Drawing for the job (mm, zero at the part's lowest x, y, z). A direction names the side the tool comes from. Round coordinates to 2 decimals unless told otherwise and drop trailing zeros. Write each loop counter-clockwise with the first axis right and the second up, starting at its lowest first coordinate (ties: lowest second). Pieces come first, ordered by that corner, then holes. Notation, with made-up numbers: M -13.5,48 L 20.5,48 A17 ccw 20.5,73 Z; hole C -5.5,-21 d1. An arc over 180 degrees is marked long. Use a Markdown table: item, result. Add a question column.
1) Slice it at A-A on x = 203. Write the cut outline in (y, z), plus the area to 3 significant figures.
2) Slice it at C-C on y = 90. Write the cut outline in (x, z), plus the area to 3 significant figures.
3) Two-plate mould, pull along Y, no slides. Class the marked faces 1, 2, 3 and 4: released by +Y, released by -Y, zero draft, split by the parting line, or undercut.
4) Which spindle directions (+Z, -Z, +X, -X, +Y, -Y) get a long thin tool onto all of the face, cutting with end or side? Do the marked faces 5 and 6. Say none if no direction does.
5) Slice it at B-B on z = 33. Write the cut outline in (x, y).
6) Wall check: probe 1 along Y at (x, z) = (193, 52); probe 2 along X at (y, z) = (112.5, 53.5). Give the ranges that are in metal, low to high.
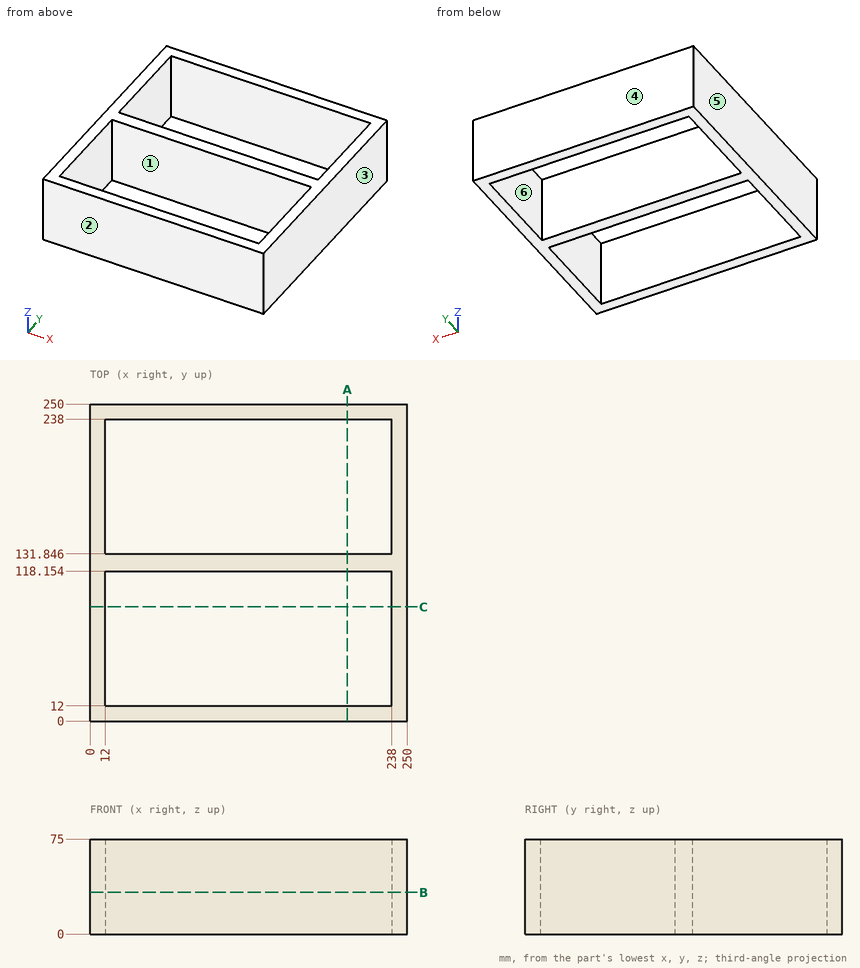
Entries:
| question | item | result |
|---|---|---|
| 1 | outline | M 0,0 L 12,0 L 12,75 L 0,75 Z; M 118.15,0 L 131.85,0 L 131.85,75 L 118.15,75 Z; M 238,0 L 250,0 L 250,75 L 238,75 Z |
| 1 | area | 2,830 mm^2 |
| 2 | outline | M 0,0 L 12,0 L 12,75 L 0,75 Z; M 238,0 L 250,0 L 250,75 L 238,75 Z |
| 2 | area | 1,800 mm^2 |
| 3 | face 1 | undercut |
| 3 | face 2 | released by -Y |
| 3 | face 3 | zero draft |
| 3 | face 4 | released by +Y |
| 4 | face 5 | +Z, -Z, -X, +Y, -Y |
| 4 | face 6 | +Z, -Z |
| 5 | outline | M 0,0 L 250,0 L 250,250 L 0,250 Z; hole M 12,12 L 238,12 L 238,118.15 L 12,118.15 Z; hole M 12,131.85 L 238,131.85 L 238,238 L 12,238 Z |
| 6 | probe 1 | y = 0 to 12, 118.15 to 131.85, 238 to 250 |
| 6 | probe 2 | x = 0 to 12, 238 to 250 |
